```python
from build123d import *

# Parameters (mm, degrees)
F1_W      = 170
F1_H      = 582.11
F2_DEPTH  = 42
F3_W      = 154
F3_H      = 566.11
F4_DEPTH  = 6
F8_R      = 5
F9_R      = 0.8
F7_W      = 46
F7_H      = 8
F10_DEPTH = 178
F11_R     = 2
F15_DEPTH = 25
F17_DEPTH = 25


with BuildPart() as f2:
    # F1 (on Front) → F2 (new body)
    with BuildSketch(Plane.XZ):
        Rectangle(F1_W, F1_H)
    extrude(amount=F2_DEPTH)

    # F3 (on face) → F4 (cut)
    with BuildSketch(Plane.XZ.offset(42)):
        Rectangle(F3_W, F3_H)
    extrude(amount=-F4_DEPTH, mode=Mode.SUBTRACT)

    # F8
    f8_edges = [f2.edges().sort_by_distance(p)[0] for p in [
        (-85, -21, -291.055),
        (85, -21, -291.055),
    ]]
    fillet(f8_edges, radius=F8_R)

    # F9
    f9_edges = [f2.edges().sort_by_distance(p)[0] for p in [
        (-85, -42, 2.5),
        (-77, -42, 0),
        (77, -42, 0),
        (85, -42, 2.5),
        (0, -42, -283.055),
        (85, 0, 2.5),
        (-85, 0, 2.5),
        (0, -42, 283.055),
    ]]
    fillet(f9_edges, radius=F9_R)

    # F7 (on offset) → F10 (join, through all)
    with BuildSketch(Plane(origin=(-89, 0, 0), x_dir=(0, -1, 0), z_dir=(-1, 0, 0))):
        with Locations((23, 295.055)):
            Rectangle(F7_W, F7_H)
    extrude(amount=-F10_DEPTH)

    # F11
    f11_edges = [f2.edges().sort_by_distance(p)[0] for p in [
        (0, -46, 299.055),
        (0, 0, 299.055),
        (-89, -23, 299.055),
        (89, -23, 299.055),
        (-89, -46, 295.055),
        (89, -46, 295.055),
        (89, 0, 295.055),
        (-89, 0, 295.055),
        (-89, -23, 291.055),
        (0, -46, 291.055),
        (89, -23, 291.055),
    ]]
    fillet(f11_edges, radius=F11_R)

    # F14 (on offset) → F15 (join)
    with BuildSketch(Plane.XY.offset(100)):
        with BuildLine():
            Line((-32.25, 1.2), (-32.25, 0))
            Line((-32.25, 0), (-18.25, 0))
            Line((-18.25, 0), (-18.25, 18))
            ThreePointArc((-18.25, 18), (0, 36.25), (18.25, 18))
            Line((18.25, 18), (18.25, 0))
            Line((18.25, 0), (32.25, 0))
            Line((32.25, 0), (32.25, 1.2))
            Line((32.25, 1.2), (19.45, 1.2))
            Line((19.45, 1.2), (19.45, 18))
            ThreePointArc((19.45, 18), (0, 37.45), (-19.45, 18))
            Line((-19.45, 18), (-19.45, 1.2))
            Line((-19.45, 1.2), (-32.25, 1.2))
        make_face()
    extrude(amount=F15_DEPTH)

    # F16 (on offset) → F17 (join)
    with BuildSketch(Plane.XY.offset(-100)):
        with BuildLine():
            Line((32.25, 1.2), (19.45, 1.2))
            Line((19.45, 1.2), (19.45, 18))
            ThreePointArc((19.45, 18), (0, 37.45), (-19.45, 18))
            Line((-19.45, 18), (-19.45, 1.2))
            Line((-19.45, 1.2), (-32.25, 1.2))
            Line((-32.25, 1.2), (-32.25, 0))
            Line((-32.25, 0), (-18.25, 0))
            Line((-18.25, 0), (-18.25, 18))
            ThreePointArc((-18.25, 18), (0, 36.25), (18.25, 18))
            Line((18.25, 18), (18.25, 0))
            Line((18.25, 0), (32.25, 0))
            Line((32.25, 0), (32.25, 1.2))
        make_face()
    extrude(amount=F17_DEPTH)


solid = f2.part
```
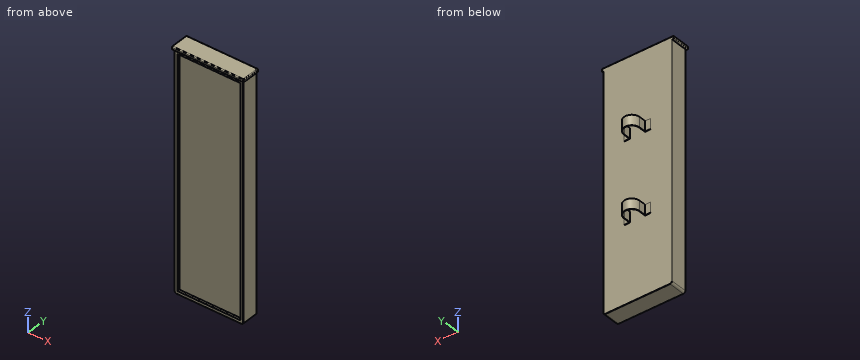
Geometry: final body of the model. Coordinates: model frame, mm. Give positions to 0.01 mm unless a question says otherwise; leave off trailing zeros. Write each loop counter-clockwise with the first axis right and the second up, starting at its lowest first coordinate (ties: lowest second). Pieces come first, ordered by that corner, then holes.
1. Line query: probe 1 along X at (y, z) = (-41.5, -242.5); probe 2 along X at (y, z) = (-8.5, -178.5); probe 3 along Y at (x, z) = (-30, 70). Output: solid intervals per line, ascending.
2. Section query B-B, the plane z = 117.5. Return loops of the section in (x, y).
3. Section query A-A, the plane x = 0. Return loops of the section in (y, z) (3 decimals).
4. Section query C-C, the plane x = 65.5. Return loops of the section in (y, z) (3 decimals), then the cut area to 3 significant figures.
5. Pin query (flat end, axial travel): P1, Ø3, axis at x = -40.5, z = 231, coming from the -Y side; P2, Ø13.5, axis at y = 12.5, z = 118, coming from the +X side; P3, Ø6.5, axis at x = 23, z = 117, coming from the +Y side. Return the tip coordinate at first contact, or that it passes through.
Computed:
1. probe 1: x = -84.94 to -77.06, 77.06 to 84.94
1. probe 2: x = -85 to 85
1. probe 3: y = -36 to 0
2. outline: (-85, -41.2) arc R0.8 ccw to (-84.2, -42) - (-77.8, -42) arc R0.8 ccw to (-77, -41.2) - (-77, -36) - (77, -36) - (77, -41.2) arc R0.8 ccw to (77.8, -42) - (84.2, -42) arc R0.8 ccw to (85, -41.2) - (85, -0.8) arc R0.8 ccw to (84.2, 0) - (32.25, 0) - (32.25, 1.2) - (19.45, 1.2) - (19.45, 18) arc R19.45 ccw to (-19.45, 18) - (-19.45, 1.2) - (-32.25, 1.2) - (-32.25, 0) - (-84.2, 0) arc R0.8 ccw to (-85, -0.8) - close; hole (-18.25, 0) - (18.25, 0) - (18.25, 18) arc R18.25 ccw to (-18.25, 18) - close
3. outline: (-46, 293.055) arc R2 ccw to (-44, 291.055) - (-42, 291.055) - (-42, 283.855) arc R0.8 ccw to (-41.2, 283.055) - (-36, 283.055) - (-36, -283.055) - (-41.2, -283.055) arc R0.8 ccw to (-42, -283.855) - (-42, -290.255) arc R0.8 ccw to (-41.2, -291.055) - (-0.8, -291.055) arc R0.8 ccw to (0, -290.255) - (0, 297.055) arc R2 ccw to (-2, 299.055) - (-44, 299.055) arc R2 ccw to (-46, 297.055) - close; (36.25, -100) - (37.45, -100) - (37.45, -75) - (36.25, -75) - close; (36.25, 100) - (37.45, 100) - (37.45, 125) - (36.25, 125) - close
4. outline: (-46, 293.055) arc R2 ccw to (-44, 291.055) - (-42, 291.055) - (-42, 283.855) arc R0.8 ccw to (-41.2, 283.055) - (-36, 283.055) - (-36, -283.055) - (-41.2, -283.055) arc R0.8 ccw to (-42, -283.855) - (-42, -290.255) arc R0.8 ccw to (-41.2, -291.055) - (-0.8, -291.055) arc R0.8 ccw to (0, -290.255) - (0, 297.055) arc R2 ccw to (-2, 299.055) - (-44, 299.055) arc R2 ccw to (-46, 297.055) - close
4. area: 21,400 mm2
5. P1: stops at y = -36
5. P2: stops at x = 19.45
5. P3: stops at y = 1.2
